The model under review builds one solid part; all positions refer to its coordinate system, in mm. A direction names the side the tool comes from. Round coordinates to 2 decimals unless told otherwise and drop trailing zeros. Write each loop counter-clockwise with the first axis right and the second up, starting at its lowest first coordinate (ties: lowest second). Pieces come first, ordered by that corner, then holes. Notation, with made-up numbers: (46, 13.25) -> (67, 13.25) arc R16 ccw to (67, 41.25) -> close; hole circle Ø5 at (7.5, 7.25). An arc over 180 degrees is marked (long way). Return JSON: item names as keys, results as strings. Group by question number.
1. Clearance check with a flat-ended pin moving along its axis: P1, Ø1.3, axis at x = -16.5, z = -34.5, coming from the +Y side. State where the tip first meets the part, or that it passes through.
2. Mouldability with a two-part tool opening along Z and no side actions: class faces 1 (the cylindrical face through (16.46, 3.48, -32.95)), 2 (the cylindrical face through (32.248, 2.535, -49.287)), 3 (the flat face through (0, 2, 50)), 4 (the cylindrical face through (-15.54, 3.48, -32.95)) as pulls with the +Z half, pulls with the -Z half, needs draft (parallel to the pull), parting line crosses it, or undercut.
3. For line 1 along Z through (x, y) = (-16, 3.5); line 2 along X through (y, z) = (3.85, 35); line 3 along X through (y, z) = (3.6, -35.5), list the stretches that pass through material, from the lowest coordinate up. Write a range as from..to.
4. Take a section at A-A, the plane x = -16. Write out the cut boundary in (y, z), then the cut area to 3 significant figures.
5. Take a section at B-B, the plane z = -35. Write out the cut boundary in (x, y), then the cut area to 3 significant figures.
6. Tool access review of faces 5 (the cylindrical face through (16.46, 3.48, 37.05)), 6 (the cylindrical face through (32.248, 2.535, 49.287)): name each direction out of +Z, -Z, +X, -X, +Y, -Y from which nothing blocks a thin tool from reaching the whole face with its end or side.
from build123d import *

# Parameters (mm, degrees)
SKETCH1_W                 = 66
SKETCH1_H                 = 100
BOSS_EXTRUDE1_DEPTH       = 5
F_4_0MM_DOWEL_HOLE1_D     = 4.2
F_4_0MM_DOWEL_HOLE1_DEPTH = 3
FILLET1_R                 = 2.5


with BuildPart() as part:
    # Sketch1 → Boss-Extrude1 (new body)
    with BuildSketch(Plane(origin=(0, 0, 0), x_dir=(1, 0, 0), z_dir=(0, 1, 0))):
        Rectangle(SKETCH1_W, SKETCH1_H)
    extrude(amount=BOSS_EXTRUDE1_DEPTH)

    # Ø4.0mm Dowel Hole1
    with Locations(Plane(origin=(0, 5, 0), x_dir=(1, 0, 0), z_dir=(0, 1, 0))):
        with Locations((-16, 35), (16, 35), (16, -35), (-16, -35)):
            Hole(F_4_0MM_DOWEL_HOLE1_D / 2, depth=F_4_0MM_DOWEL_HOLE1_DEPTH)

    # Fillet1
    fillet1_edges = [part.edges().sort_by_distance(p)[0] for p in [
        (-33, 2.5, -50),
        (33, 2.5, -50),
        (33, 2.5, 50),
        (-33, 2.5, 50),
    ]]
    fillet(fillet1_edges, radius=FILLET1_R)


solid = part.part
Output:
{
 "1": {"P1": "stops at y = 2"},
 "2": {"face 1": "undercut", "face 2": "pulls with the -Z half", "face 3": "pulls with the +Z half", "face 4": "undercut"},
 "3": {"line 1": "z = -50..-37.1, -32.9..32.9, 37.1..50", "line 2": "x = -33..-18.1, -13.9..13.9, 18.1..33", "line 3": "x = -33..-18.04, -13.96..13.96, 18.04..33"},
 "4": {"outline": "(0, -50) -> (5, -50) -> (5, -37.1) -> (2, -37.1) -> (2, -32.9) -> (5, -32.9) -> (5, 32.9) -> (2, 32.9) -> (2, 37.1) -> (5, 37.1) -> (5, 50) -> (0, 50) -> close", "area": "475 mm^2"},
 "5": {"outline": "(-33, 0) -> (33, 0) -> (33, 5) -> (18.1, 5) -> (18.1, 2) -> (13.9, 2) -> (13.9, 5) -> (-13.9, 5) -> (-13.9, 2) -> (-18.1, 2) -> (-18.1, 5) -> (-33, 5) -> close", "area": "305 mm^2"},
 "6": {"face 5": "+Y", "face 6": "+Z, +X, +Y, -Y"}
}
